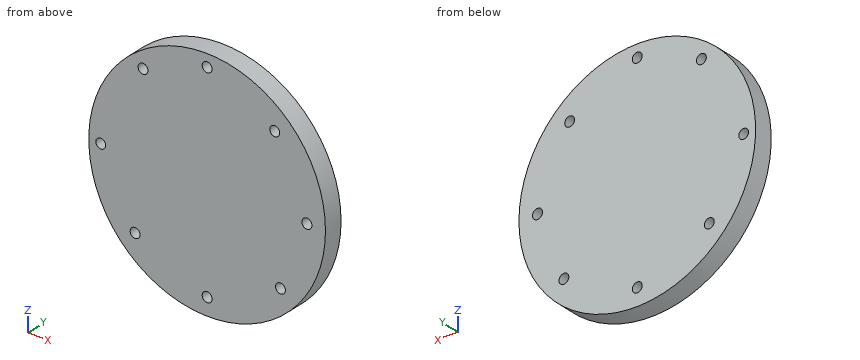
from build123d import *

# Parameters (mm, degrees)
F0_R     = 76.2210632732
F1_DEPTH = 12.7
F2_R     = 3.1879491609
F2_R_2   = 3.1879465914
F2_R_3   = 3.2380529084
F2_R_4   = 3.1498446293
F2_R_5   = 3.1721232023
F2_R_6   = 3.1721218695
F2_R_7   = 3.1721255347
F2_R_8   = 3.1721262011
F3_DEPTH = 25.4


# Not quite as in the source:
# - a length typed as a fraction of an inch, garbled in the dataset ("3 / 203.2 mm" for 3/8 in), is restored


with BuildPart() as f1:
    # F0 (on Front) → F1 (new body)
    with BuildSketch(Plane.XZ):
        Circle(F0_R)
    extrude(amount=F1_DEPTH)

    # F2 (on Front) → F3 (cut)
    with BuildSketch(Plane.XZ):
        with Locations((0, 68.2354792953)):
            Circle(F2_R)
        with Locations((0, -65.1145204902)):
            Circle(F2_R_2)
        with Locations((64.2633512616, 0)):
            Circle(F2_R_3)
        with Locations((-68.519204855, 0)):
            Circle(F2_R_4)
        with Locations((-41.2817560136, 52.9144145548)):
            Circle(F2_R_5)
        with Locations((47.2399480641, -43.5515418649)):
            Circle(F2_R_6)
        with Locations((-46.3887788355, -44.118989259)):
            Circle(F2_R_7)
        with Locations((43.5515418649, 46.3887788355)):
            Circle(F2_R_8)
    extrude(amount=F3_DEPTH, mode=Mode.SUBTRACT)


solid = f1.part
Geometry: final body of the model. Coordinates: model frame, mm. Give positions to 0.01 mm unless a question says otherwise; leave off trailing zeros. Loops run counter-clockwise (first coordinate to the right, second up) from the corner with the lowest first, then second, coordinate; pieces in that order, holes last. Notation, with made-up numbers: M -18,56 L 4,56 A24 cw 4,82 Z; hole C 18.5,-10.5 d1. An arc over 180 degrees is marked long. Put each result on its own line as item: value. Start each with the question number.
1) Cut plane D-D (x = -24). Output: boundary loops of the cut face in (y, z).
2) Ray query, line 1 along Z through (x, y) = (0, -9.5); line 2 along X through (y, z) = (-9.25, -0.5); line 3 along Z through (x, y) = (-2, -4.5). Return the intervals inside material, ascending.
3) Cut plane C-C (y = -5.5). Give the number of separate pieces and of enclosed holes in the cut face, then the cut area to 3 significant figures.
4) Cut plane B-B (x = 0). Output: boundary loops of the cut face in (y, z).
5) Contact query for flat-ended pins moving along their axis: pin 1 (5 mm diameter, centred on x = 43.55, z = 46.39, fed in from -Y); pin 2 (1.5 mm diameter, centred on x = -49.5, y = -2.5, fed in from -Z); pin 3 (4 mm diameter, centred on y = -8.5, z = -59, fed in from -X); pin 4 (2 mm diameter, centred on x = -15, y = -10.5, fed in from -Z). Output: stop coordinate, or through.
6) Cut plane A-A (z = 0). Output: boundary loops of the cut face in (x, y).
Verdict:
1. outline: M -12.7,-72.34 L 0,-72.34 L 0,72.34 L -12.7,72.34 Z
2. line 1: -76.22 to -68.3, -61.93 to 65.05, 71.42 to 76.22
2. line 2: -76.22 to -71.63, -65.41 to 61.06, 67.46 to 76.22
2. line 3: -76.19 to -67.6, -62.63 to 65.75, 70.72 to 76.19
3. separate pieces: 1
3. enclosed holes: 8
3. area: 18,000 mm2
4. outline: M -12.7,-76.22 L 0,-76.22 L 0,-68.3 L -12.7,-68.3 Z; M -12.7,-61.93 L 0,-61.93 L 0,65.05 L -12.7,65.05 Z; M -12.7,71.42 L 0,71.42 L 0,76.22 L -12.7,76.22 Z
5. pin 1: through
5. pin 2: z = -58.59
5. pin 3: x = -50.6
5. pin 4: z = -74.92
6. outline: M -76.22,-12.7 L -71.67,-12.7 L -71.67,0 L -76.22,0 Z; M -65.37,-12.7 L 61.03,-12.7 L 61.03,0 L -65.37,0 Z; M 67.5,-12.7 L 76.22,-12.7 L 76.22,0 L 67.5,0 Z
